Input: part model. Units: mm. Frame: model coordinates. A direction names the side the tool comes from. Give positions to 0.01 mm unless a question says otherwise; leave off trailing zeros. Loops run counter-clockwise (first coordinate to the right, second up) from the corner with the lowest first, then second, coordinate; pieces in that order, holes last. Notation, with made-up numbers: (77.25, 11) -> (81.25, 11) arc R14 ccw to (81.25, 26) -> close; hole circle Ø2 at (-9.75, 35). An arc over 180 degrees is marked (long way). Answer as a JSON object with one key per item and string values.
```python
from build123d import *

# Parameters (mm, degrees)
F0_W        = 104
F0_H        = 104
F0_R        = 1.5
F0_R_2      = 2.5
F2_DEPTH    = 10
F2_FACE_W   = 104
F2_FACE_H   = 104
F2_FACE_R   = 1.5
F2_FACE_R_2 = 2.5
F3_DEPTH    = 25
F4_R        = 1


with BuildPart() as f2:
    # F0 (on Front) → F2 (new body)
    with BuildSketch(Plane.XZ):
        with Locations((1.0205563903, -3.0722830892)):
            Rectangle(F0_W, F0_H)
        with Locations((-47.2263507545, -50.8087884027)):
            Circle(F0_R, mode=Mode.SUBTRACT)
        with Locations((-40.6989715993, -43.9550094306)):
            Circle(F0_R_2, mode=Mode.SUBTRACT)
        with Locations((49.0661785007, -49.9558521996)):
            Circle(F0_R, mode=Mode.SUBTRACT)
        with Locations((41.4574928582, -43.9577177167)):
            Circle(F0_R_2, mode=Mode.SUBTRACT)
        with Locations((-47.2263507545, 45.0361557305)):
            Circle(F0_R, mode=Mode.SUBTRACT)
        with Locations((49.0661785007, 45.0242571533)):
            Circle(F0_R, mode=Mode.SUBTRACT)
    extrude(amount=F2_DEPTH)

    # F1 (on Front) + F2_face (on face) → F3 (cut)
    with BuildSketch(Plane.XZ):
        with BuildLine():
            Line((37.4257260145, 39.1947293328), (-36.9051963783, 39.1947293328))
            ThreePointArc((-36.9051963783, 39.1947293328), (-37.7897278988, 38.9884974308), (-38.4918408014, 38.4123333221))
            Line((-38.4918408014, 38.4123333221), (-43.5660880328, 31.8001456637))
            ThreePointArc((-43.5660880328, 31.8001456637), (-43.873287432, 31.2254690241), (-43.9794436097, 30.5825416744))
            Line((-43.9794436097, 30.5825416744), (-43.9794436097, -29.8682280959))
            ThreePointArc((-43.9794436097, -29.8682280959), (-43.7905206373, -30.7167562333), (-43.2594436097, -31.4049779128))
            Line((-43.2594436097, -31.4049779128), (-24.0500708974, -47.4049779128))
            ThreePointArc((-24.0500708974, -47.4049779128), (-23.4506957449, -47.7488529433), (-22.7700708974, -47.8682280959))
            Line((-22.7700708974, -47.8682280959), (25.2299291026, -47.8682280959))
            ThreePointArc((25.2299291026, -47.8682280959), (25.8975098604, -47.7764802387), (26.4967279793, -47.4682280959))
            Line((26.4967279793, -47.4682280959), (45.3353493779, -31.0333157505))
            ThreePointArc((45.3353493779, -31.0333157505), (45.8412136858, -30.3539983577), (46.0205563903, -29.5262260386))
            Line((46.0205563903, -29.5262260386), (46.0205563903, 32.097225442))
            ThreePointArc((46.0205563903, 32.097225442), (45.815861416, 32.9786333298), (45.2436765256, 33.6796214527))
            Line((45.2436765256, 33.6796214527), (38.6488461498, 38.7771253435))
            ThreePointArc((38.6488461498, 38.7771253435), (38.071948878, 39.0874511853), (37.4257260145, 39.1947293328))
        make_face()
    with BuildSketch(Plane(origin=(1.0231641347, -10, -2.9239537764), x_dir=(1, 0, 0), z_dir=(0, -1, 0))):
        with Locations((-0.0026077444, -0.1483293127)):
            Rectangle(F2_FACE_W, F2_FACE_H)
        with Locations((-48.2495148892, -47.8848346262)):
            Circle(F2_FACE_R, mode=Mode.SUBTRACT)
        with Locations((-41.7221357341, -41.0310556542)):
            Circle(F2_FACE_R_2, mode=Mode.SUBTRACT)
        with Locations((48.0430143659, -47.0318984232)):
            Circle(F2_FACE_R, mode=Mode.SUBTRACT)
        with Locations((40.4343287234, -41.0337639403)):
            Circle(F2_FACE_R_2, mode=Mode.SUBTRACT)
        with Locations((-48.2495148892, 47.9601095069)):
            Circle(F2_FACE_R, mode=Mode.SUBTRACT)
        with Locations((48.0430143659, 47.9482109297)):
            Circle(F2_FACE_R, mode=Mode.SUBTRACT)
    extrude(amount=F3_DEPTH, mode=Mode.SUBTRACT)

    # F4
    f4_edges = [f2.edges().sort_by_distance(p)[0] for p in [
        (-50.979444, -5, 48.927717),
        (-50.979444, -10, -3.072283),
        (1.020556, -10, 48.927717),
        (-50.979444, -5, -55.072283),
        (1.020556, -10, -55.072283),
        (53.020556, -10, -3.072283),
        (53.020556, -5, 48.927717),
        (53.020556, -5, -55.072283),
    ]]
    fillet(f4_edges, radius=F4_R)


solid = f2.part
```
Q1. Draft query along X for faces 1 (the flat face through (1, -10, 42)), 2 (the flat face through (53.021, -4, -4)), 3 (the cylindrical face through (-38.39, -4.93, -44.91)). Return one class per face: +X half, -X half, draft (parallel to the pull), parting line (faces both ways), or undercut.
Evaluation:
{"face 1": "draft", "face 2": "+X half", "face 3": "undercut"}
Q2. Section C-C, the plane y = -2.75. Give the number of separate pieces and of enclosed holes in the cut face, then the cut area to 3 significant figures.
Evaluation:
{"separate pieces": "1", "enclosed holes": "7", "area": "3,310 mm2"}
Q3. Access query for faces 4 (the flat face through (0, -4, 48.928)), 5 (the flat face through (1, -5, -47.868)). Directions: +Z, -Z, +X, -X, +Y, -Y. A direction counts if a zero-diameter tool reaches every point of the face in a straight line with its end or side. Return the directions, or none.
Evaluation:
{"face 4": "+Z, +X, -X, +Y, -Y", "face 5": "+Y, -Y"}
Q4. Section B-B, the plane x = 18. Return the cut outline in (y, z), then the cut area to 3 significant figures.
Evaluation:
{"outline": "(-10, -54.07) arc R1 ccw to (-9, -55.07) -> (0, -55.07) -> (0, -47.87) -> (-10, -47.87) -> close; (-10, 39.19) -> (0, 39.19) -> (0, 48.93) -> (-9, 48.93) arc R1 ccw to (-10, 47.93) -> close", "area": "169 mm2"}
Q5. Ray query, line 1 along Z through (x, y) = (-22, -3.5); line 2 along Z through (x, y) = (40.5, -4.25); line 3 along X through (y, z) = (-6.75, 22). Return the intervals inside material, ascending.
Evaluation:
{"line 1": "z = -55.07 to -47.87, 39.19 to 48.93", "line 2": "z = -55.07 to -46.27, -41.65 to -35.25, 37.35 to 48.93", "line 3": "x = -50.98 to -43.98, 46.02 to 53.02"}
Q6. Section A-A, the plane z = 28. Return the cut outline in (x, y), then the cut area to 3 significant figures.
Evaluation:
{"outline": "(-50.98, -9) arc R1 ccw to (-49.98, -10) -> (-43.98, -10) -> (-43.98, 0) -> (-50.98, 0) -> close; (46.02, -10) -> (52.02, -10) arc R1 ccw to (53.02, -9) -> (53.02, 0) -> (46.02, 0) -> close", "area": "140 mm2"}
